Here's the drawing with two shaded views (mm, measured from the low corner). I have some questions. A direction names the side the tool comes from. Give positions to 0.01 mm unless a question says otherwise; leave off trailing zeros. Loops run counter-clockwise (first coordinate to the right, second up) from the corner with the lowest first, then second, coordinate; pieces in that order, holes last. Notation, with made-up numbers: (30, 6.25) -> (45, 6.25) arc R16 cw to (45, 16.25) -> close; hole circle Ø4 at (-39.5, 10). An arc over 180 degrees is marked (long way). Put each result on its own line as item: value.
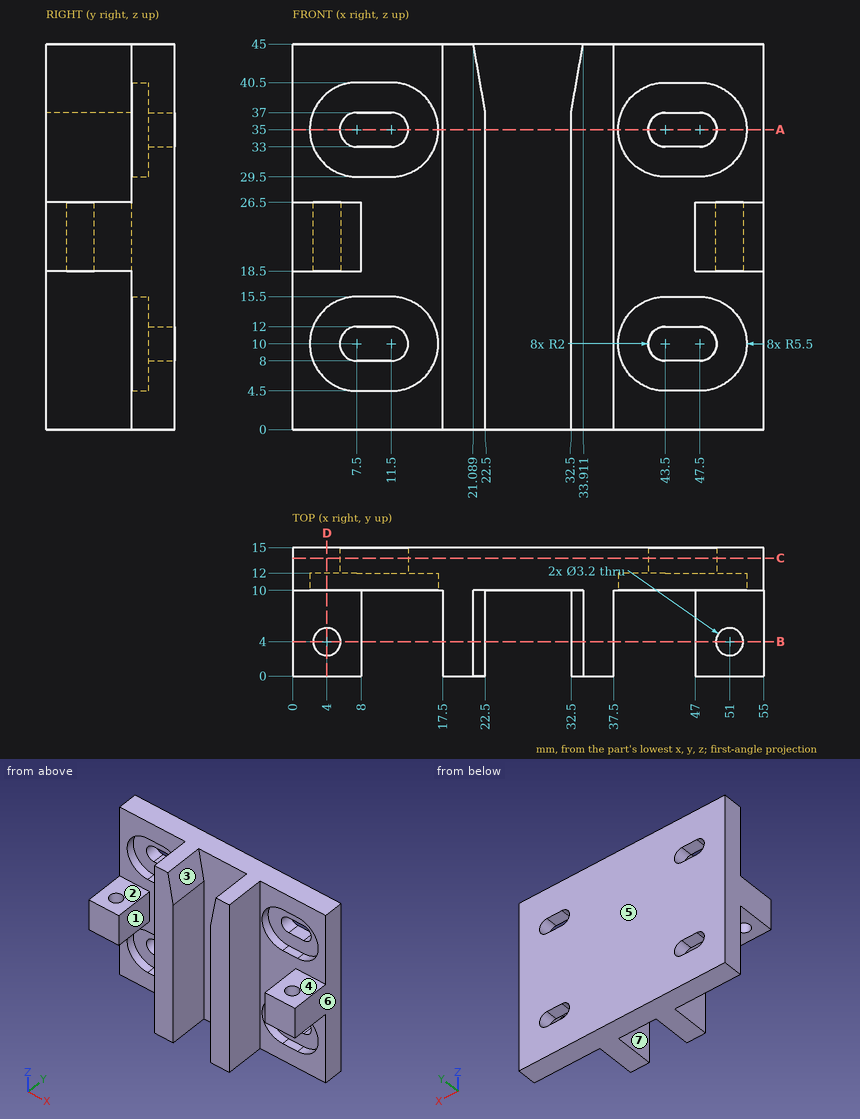
1. If we section it at C-C (y = 13.75): List the corners of the cut face in (x, z) for me, then the cut area to 3 significant figures.
Recorded:
outline: (0, 0) -> (55, 0) -> (55, 45) -> (0, 45) -> close; hole (7.5, 8) -> (11.5, 8) arc R2 ccw to (11.5, 12) -> (7.5, 12) arc R2 ccw to start; hole (7.5, 33) -> (11.5, 33) arc R2 ccw to (11.5, 37) -> (7.5, 37) arc R2 ccw to start; hole (43.5, 8) -> (47.5, 8) arc R2 ccw to (47.5, 12) -> (43.5, 12) arc R2 ccw to start; hole (43.5, 33) -> (47.5, 33) arc R2 ccw to (47.5, 37) -> (43.5, 37) arc R2 ccw to start
area: 2,360 mm^2
2. If we section it at D-D (x = 4): List the corners of the cut face in (y, z) for me.
Recorded:
outline: (0, 18.5) -> (2.4, 18.5) -> (2.4, 26.5) -> (0, 26.5) -> close; (5.6, 18.5) -> (10, 18.5) -> (10, 14.24) -> (12, 14.24) -> (12, 5.76) -> (10, 5.76) -> (10, 0) -> (15, 0) -> (15, 45) -> (10, 45) -> (10, 39.24) -> (12, 39.24) -> (12, 30.76) -> (10, 30.76) -> (10, 26.5) -> (5.6, 26.5) -> close
3. I'm going to push flat-ended pins straight in: pin 1 (6.5 mm diameter, centred on x = 2, y = 4, fed in from -Z); pin 2 (5 mm diameter, centred on x = 48, z = 35, fed in from -Y); pin 3 (9 mm diameter, centred on x = 43.5, z = 8.5, fed in from -Y). Where does each tip first touch, or does it pass through?
Recorded:
pin 1: stops at z = 18.5
pin 2: stops at y = 12
pin 3: stops at y = 10
4. If we section it at B-B (y = 4): List the corners of the cut face in (x, z) for me.
Recorded:
outline: (0, 18.5) -> (2.4, 18.5) -> (2.4, 26.5) -> (0, 26.5) -> close; (5.6, 18.5) -> (8, 18.5) -> (8, 26.5) -> (5.6, 26.5) -> close; (17.5, 0) -> (22.5, 0) -> (22.5, 37) -> (21.09, 45) -> (17.5, 45) -> close; (32.5, 0) -> (37.5, 0) -> (37.5, 45) -> (33.91, 45) -> (32.5, 37) -> close; (47, 18.5) -> (49.4, 18.5) -> (49.4, 26.5) -> (47, 26.5) -> close; (52.6, 18.5) -> (55, 18.5) -> (55, 26.5) -> (52.6, 26.5) -> close
5. Thinking about a two-plate mould opening in X: for the marked faces 5, 6 and 7, which applies, pulls with the +X half, pulls with the -X half, needs draft (parallel to the pull), parting line crosses it, or undercut?
Recorded:
face 5: needs draft
face 6: pulls with the +X half
face 7: undercut
6. For the marked faces 1, 2, 3 and 4, which set-ups out of +Z, -Z, +X, -X, +Y, -Y let a thin tool reach every point of the face, with its end or its side?
Recorded:
face 1: +Z, -Z, -Y
face 2: +Z, -X, -Y
face 3: +Z, -Y
face 4: +Z, +X, -Y
7. I need wall thicknesses on line 1 (Z direction, x = 44, y = 10.5); line 2 (X direction, y = 2, z = 22); line 3 (Y direction, x = 51, z = 23.5). Which ranges of each line are inside material? Lowest first, please.
Recorded:
line 1: z = 0 to 4.5, 15.5 to 29.5, 40.5 to 45
line 2: x = 0 to 8, 17.5 to 22.5, 32.5 to 37.5, 47 to 55
line 3: y = 0 to 2.4, 5.6 to 15
8. If we section it at A-A (z = 35): List the corners of the cut face in (x, y) for me.
Recorded:
outline: (0, 10) -> (2, 10) -> (2, 12) -> (5.5, 12) -> (5.5, 15) -> (0, 15) -> close; (13.5, 12) -> (17, 12) -> (17, 10) -> (17.5, 10) -> (17.5, 0) -> (22.5, 0) -> (22.5, 10) -> (32.5, 10) -> (32.5, 0) -> (37.5, 0) -> (37.5, 10) -> (38, 10) -> (38, 12) -> (41.5, 12) -> (41.5, 15) -> (13.5, 15) -> close; (49.5, 12) -> (53, 12) -> (53, 10) -> (55, 10) -> (55, 15) -> (49.5, 15) -> close
